from build123d import *

# Parameters (mm, degrees)
SKETCH1_W             = 78.74
SKETCH1_H             = 66.04
BOSS_EXTRUDE1_DEPTH   = 5.08
SKETCH2_R             = 4.699
SKETCH2_R_2           = 2.7686
CUT_EXTRUDE1_DEPTH    = 5.08
F_4_CLEARANCE_HOLE1_D = 3.2512


with BuildPart() as part:
    # Sketch1 → Boss-Extrude1 (new body)
    with BuildSketch(Plane(origin=(0, 0, 0), x_dir=(1, 0, 0), z_dir=(0, 1, 0))):
        Rectangle(SKETCH1_W, SKETCH1_H)
    extrude(amount=BOSS_EXTRUDE1_DEPTH)

    # Sketch2 → Cut-Extrude1 (cut)
    with BuildSketch(Plane(origin=(0, 5.08, 0), x_dir=(1, 0, 0), z_dir=(0, 1, 0))):
        with Locations(Location((-8.7122, 0, 0), (0, 0, 270))):
            Circle(SKETCH2_R)
        with Locations(Location((8.636, 0, 0), (0, 0, 270))):
            Circle(SKETCH2_R_2)
    extrude(amount=-CUT_EXTRUDE1_DEPTH, mode=Mode.SUBTRACT)

    # #4 Clearance Hole1 (through all)
    with Locations(Plane(origin=(0, 5.08, 0), x_dir=(1, 0, 0), z_dir=(0, 1, 0))):
        with Locations((-35.56, 29.21), (-35.56, -29.21), (35.676601494, -29.21), (35.56, 29.21)):
            Hole(F_4_CLEARANCE_HOLE1_D / 2)


solid = part.part
Can you work these out from the model? Positions are in its coordinate system, mm. Round coordinates to 2 decimals unless told otherwise and drop trailing zeros. Order: outer loops, then holes, each group sorted by start corner. A loop starts at its lowest first (then second) coordinate and runs counter-clockwise, first axis right, second up. Notation, with made-up numbers: (19, 45.5) -> (50, 45.5) arc R16 cw to (50, 58.5) -> close; hole circle Ø11 at (-39.5, 51.5). An arc over 180 degrees is marked (long way). Write each question's results on one line, items separated by ' | '. Start each with the question number.
Item 1: If we section it at C-C, the plane z = 0: Write out the boundary of the cut face in (x, y).
Item 2: Will this pin go through, and if not, where does the flat tip stop? pin 1 (2 mm diameter, centred on x = -35.56, z = -29.21, fed in from -Y).
Item 3: Please list where these lines run through material, in increasing order: L1, parallel to X at y = 2.15, z = 0; L2, parallel to X at y = 2.9, z = -29.21; L3, parallel to Z at x = -35.56, y = 3.95.
Item 4: If we section it at A-A, the plane z = -29.21: Write out the boundary of the cut face in (x, y), then the cut area to 3 significant figures.
Item 5: If we section it at B-B, the plane y = 0.85: Write out the boundary of the cut face in (x, z).
Item 6: Thinking about a two-plate mould opening in X: for faces 1 (the flat face through (-1, 5.08, 0)), 2 (the cylindrical face through (36.029, 2.504, 30.797)), 3 (the flat face through (39.37, 3, 0)), 4 (the flat face through (-39.37, 3, 0)), which applies, +X half, -X half, draft (parallel to the pull), parting line (faces both ways), or undercut?
Results:
1) outline: (-39.37, 0) -> (-13.41, 0) -> (-13.41, 5.08) -> (-39.37, 5.08) -> close; (-4.01, 0) -> (5.87, 0) -> (5.87, 5.08) -> (-4.01, 5.08) -> close; (11.4, 0) -> (39.37, 0) -> (39.37, 5.08) -> (11.4, 5.08) -> close
2) pin 1: passes through
3) L1: x = -39.37 to -13.41, -4.01 to 5.87, 11.4 to 39.37 | L2: x = -39.37 to -37.19, -33.93 to 33.93, 37.19 to 39.37 | L3: z = -33.02 to -30.84, -27.58 to 27.58, 30.84 to 33.02
4) outline: (-39.37, 0) -> (-37.19, 0) -> (-37.19, 5.08) -> (-39.37, 5.08) -> close; (-33.93, 0) -> (33.93, 0) -> (33.93, 5.08) -> (-33.93, 5.08) -> close; (37.19, 0) -> (39.37, 0) -> (39.37, 5.08) -> (37.19, 5.08) -> close | area: 367 mm2
5) outline: (-39.37, -33.02) -> (39.37, -33.02) -> (39.37, 33.02) -> (-39.37, 33.02) -> close; hole circle Ø3.25 at (-35.56, -29.21); hole circle Ø3.25 at (-35.56, 29.21); hole circle Ø9.4 at (-8.71, 0); hole circle Ø5.54 at (8.64, 0); hole circle Ø3.25 at (35.56, -29.21); hole circle Ø3.25 at (35.68, 29.21)
6) face 1: draft | face 2: undercut | face 3: +X half | face 4: -X half
